Here's how the part is built. I have some questions about the finished solid (model axes, mm). Face numbers are marked on the shaded views. A direction names the side the tool comes from. Give positions to 0.01 mm unless a question says otherwise; leave off trailing zeros. Write each loop counter-clockwise with the first axis right and the second up, starting at its lowest first coordinate (ties: lowest second). Pieces come first, ordered by that corner, then holes. Notation, with made-up numbers: (83.5, 13) - (140.5, 13) arc R30 cw to (140.5, 51) - close; hole circle Ø5 at (40, 87). An arc over 180 degrees is marked (long way). Use a Markdown table: item, result.
```python
from build123d import *

# Parameters (mm, degrees)
SKETCH_1_W      = 4
SKETCH_1_H      = 6
SKETCH_1_R      = 1
EXTRUDE_1_DEPTH = 1
SKETCH_2_W      = 3
SKETCH_2_H      = 6
SKETCH_2_R      = 1
SKETCH_2_W_2    = 3.5
EXTRUDE_2_DEPTH = 1
FILLET_1_R      = 1


with BuildPart() as part:
    # 草图1 → 凸台-拉伸1 (new body)
    with BuildSketch(Plane.XY):
        Rectangle(SKETCH_1_W, SKETCH_1_H)
        Circle(SKETCH_1_R, mode=Mode.SUBTRACT)
    extrude(amount=EXTRUDE_1_DEPTH)

    # 草图2 → 凸台-拉伸2 (add)
    # profile 1 of 2: a face of its own
    with BuildSketch(Plane(origin=(2, 0, 0), x_dir=(0, 0, -1), z_dir=(1, 0, 0))):
        with Locations((-2.5, 0)):
            Rectangle(SKETCH_2_W, SKETCH_2_H)
        with Locations(Location((-2.5, 0, 0), (0, 0, 90))):
            Circle(SKETCH_2_R, mode=Mode.SUBTRACT)
    # profile 2 of 2: a face of its own
    with BuildSketch(Plane(origin=(2, 0, 0), x_dir=(0, 0, -1), z_dir=(1, 0, 0))):
        with Locations((0.75, 0)):
            Rectangle(SKETCH_2_W_2, SKETCH_2_H)
    extrude(amount=EXTRUDE_2_DEPTH)

    # 圆角1
    fillet_1_edges = [part.edges().sort_by_distance(p)[0] for p in [
        (-2, -3, 0.5),
        (-2, 3, 0.5),
    ]]
    fillet(fillet_1_edges, radius=FILLET_1_R)

    # 镜向1: part across plane


with BuildPart() as part_1:
    add(part.part)
    add(part.part.mirror(Plane(origin=(3, 0, -2.5), x_dir=(1, 0, 0), z_dir=(0, 0, 1))))


solid = part_1.part
```
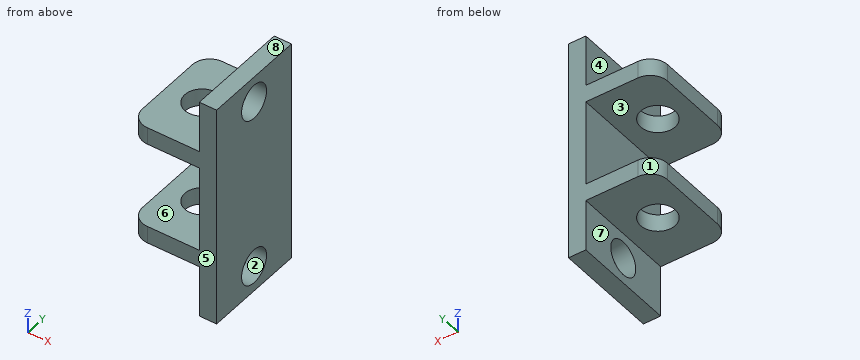
Item 1: If we section it at B-B, the plane z = -7.5: Write out the boundary of the cut face in (x, y).
Values:
| item | result |
|---|---|
| outline | (2, -3) - (3, -3) - (3, -1) - (2, -1) - close; (2, 1) - (3, 1) - (3, 3) - (2, 3) - close |
Item 2: I need wall thicknesses on line 1 along Z through (x, y) = (2.45, 0); line 2 along Z through (x, y) = (-0.5, -1.4); line 3 along Y through (x, z) = (0, -5.2). Which ranges of each line are inside material? Lowest first, please. Write a range as [from, to].
Values:
| item | result |
|---|---|
| line 1 | z = [-9, -8.5], [-6.5, 1.5], [3.5, 4] |
| line 2 | z = [-6, -5], [0, 1] |
| line 3 | y = [-3, -1], [1, 3] |
Item 3: Thinking about a two-plate mould opening in Y: for the marked faces 1, 2 and 3, which applies, +Y half, -Y half, draft (parallel to the pull), parting line (faces both ways), or undercut?
Values:
| item | result |
|---|---|
| face 1 | +Y half |
| face 2 | undercut |
| face 3 | draft |
Item 4: If we section it at C-C, the plane y = 0: Write out the boundary of the cut face in (x, z), plus the area to 3 significant figures.
Values:
| item | result |
|---|---|
| outline | (-2, -6) - (-1, -6) - (-1, -5) - (-2, -5) - close; (-2, 0) - (-1, 0) - (-1, 1) - (-2, 1) - close; (1, -6) - (2, -6) - (2, -6.5) - (3, -6.5) - (3, 1.5) - (2, 1.5) - (2, 1) - (1, 1) - (1, 0) - (2, 0) - (2, -5) - (1, -5) - close; (2, -9) - (3, -9) - (3, -8.5) - (2, -8.5) - close; (2, 3.5) - (3, 3.5) - (3, 4) - (2, 4) - close |
| area | 13.0 mm2 |
Item 5: For the marked faces 4, 5, 6, 7 and 8, which set-ups out of +Z, -Z, +X, -X, +Y, -Y let a thin tool reach every point of the face, with its end or its side?
Values:
| item | result |
|---|---|
| face 4 | +Z, -X, +Y, -Y |
| face 5 | +Z, -Z, +X, -X, -Y |
| face 6 | -X, +Y, -Y |
| face 7 | -Z, -X, +Y, -Y |
| face 8 | +Z, +X, -X, +Y, -Y |
Item 6: If we section it at D-D, the plane y = 1.8: Write out the boundary of the cut face in (x, z), plus the area to 3 significant figures.
Values:
| item | result |
|---|---|
| outline | (-2, -6) - (2, -6) - (2, -9) - (3, -9) - (3, 4) - (2, 4) - (2, 1) - (-2, 1) - (-2, 0) - (2, 0) - (2, -5) - (-2, -5) - close |
| area | 21.0 mm2 |
Item 7: Will these pins go through, and if not, where does the flat tip stop? pin 1 Ø3 at (x, y) = (-0.5, 1.5) entering from +Z; pin 2 Ø2.5 at (x, y) = (0, 0) entering from -Z; pin 3 Ø2.5 at (y, z) = (0, -7.5) entering from -X.
Values:
| item | result |
|---|---|
| pin 1 | stops at z = 1 |
| pin 2 | stops at z = -6 |
| pin 3 | stops at x = 2 |
Item 8: If we section it at A-A, the plane x = 0: Write out the boundary of the cut face in (y, z).
Values:
| item | result |
|---|---|
| outline | (-3, -6) - (-1, -6) - (-1, -5) - (-3, -5) - close; (-3, 0) - (-1, 0) - (-1, 1) - (-3, 1) - close; (1, -6) - (3, -6) - (3, -5) - (1, -5) - close; (1, 0) - (3, 0) - (3, 1) - (1, 1) - close |
